The listing builds one solid part. Answer for the finished solid, in the listing's coordinates (mm). Face numbers are marked on the shaded views. A direction names the side the tool comes from. Coordinates: 2 decimals unless noted, no trailing zeros. Write each loop counter-clockwise with the first axis right and the second up, starting at its lowest first coordinate (ties: lowest second). Pieces come first, ordered by that corner, then holes.
(1) The part is cut by section A-A on y = 41.5. Determine the outline of the cut face in (x, z).
(2) Given P1, Ø4, axis at x = -15.5, z = -48.5, coming from the -Y side; P2, Ø16, axis at y = 49.5, z = -34.5, coming from the -X side; P3, Ø2, axis at x = 29, y = -26.5, coming from the -Z side, each flat-ended and moving along its own axis, determine where each tip first touches the part or whether it passes through.
(3) Which of the six approach directions +Z, -Z, +X, -X, +Y, -Y give full straight-line access (tool end or side, diameter ignored) to the marked faces 1 and 2?
(4) The part is cut by section B-B on z = -39. Determine the outline of the cut face in (x, y).
(5) Straight lines are drawn through the part: line 1 (Y direction, x = -22, z = -18); line 2 (Z direction, x = 11, y = -1). For each, find the intervals that lie inside material, in ascending order.
from build123d import *

# Parameters (mm, degrees)
EXTRUDE_1_DEPTH           = 3
CUT_EXTRUDE_10_DEPTH      = 76.423640864
CUT_EXTRUDE_10_DEPTH_BACK = 3
SKETCH_9_W                = 95.828885904
SKETCH_9_H                = 3
EXTRUDE_2_DEPTH           = 20
SKETCH_10_W               = 95.828885904
SKETCH_10_H               = 3
EXTRUDE_3_DEPTH           = 60


with BuildPart() as part:
    # 草图1 → 凸台-拉伸1 (new body)
    with BuildSketch(Plane.XY):
        with BuildLine():
            Line((-60, 34), (-60, -34))
            add(Edge.make_bspline(
                [(-60, -34), (0, -61.168399395), (60, -34)],
                knots=[0.841357477, 0.841357477, 0.841357477, 2.300235176, 2.300235176, 2.300235176], degree=2, weights=[1, 0.745548499, 1]))
            Line((60, -34), (60, 34))
            add(Edge.make_bspline(
                [(60, 34), (0, 61.168399395), (-60, 34)],
                knots=[3.982950131, 3.982950131, 3.982950131, 5.44182783, 5.44182783, 5.44182783], degree=2, weights=[1, 0.745548499, 1]))
        make_face()
    extrude(amount=EXTRUDE_1_DEPTH)

    # 草图7 → 切除-拉伸10 (cut, two sides: drawn at the far end of the back side and taken through both)
    with BuildSketch(Plane(origin=(0, 0, 0), x_dir=(-1, 0, 0), z_dir=(0, 0, -1)).offset(-CUT_EXTRUDE_10_DEPTH_BACK)):
        with BuildLine():
            Line((-47.914442952, 38.608895735), (-0.047490379, 38.608895735))
            Line((-0.047490379, 38.608895735), (47.914442952, 38.608895735))
            add(Edge.make_bspline(
                [(-47.914442952, 38.608895735), (0, 53.86648698), (47.914442952, 38.608895735)],
                knots=[4.161758339, 4.161758339, 4.161758339, 5.263019622, 5.263019622, 5.263019622], degree=2, weights=[0.945270908, 0.800277591, 0.945270908]))
        make_face()
    extrude(amount=CUT_EXTRUDE_10_DEPTH + CUT_EXTRUDE_10_DEPTH_BACK, mode=Mode.SUBTRACT)

    # 草图9 → 凸台-拉伸2 (add)
    with BuildSketch(Plane(origin=(0, 38.608895735, 0), x_dir=(1, 0, 0), z_dir=(0, 1, 0))):
        with Locations((0, -1.5)):
            Rectangle(SKETCH_9_W, SKETCH_9_H)
    extrude(amount=EXTRUDE_2_DEPTH)

    # 草图10 → 凸台-拉伸3 (add)
    with BuildSketch(Plane(origin=(0, 0, 0), x_dir=(-1, 0, 0), z_dir=(0, 0, -1))):
        with Locations((0, 57.108895735)):
            Rectangle(SKETCH_10_W, SKETCH_10_H)
    extrude(amount=EXTRUDE_3_DEPTH)


solid = part.part
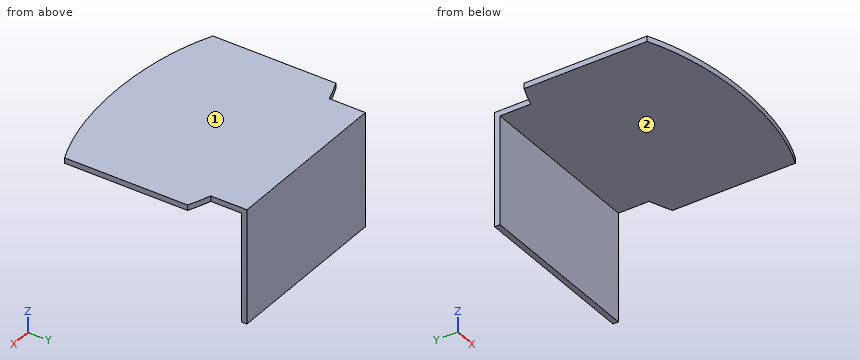
Model answer:
1. outline: (-47.91, 0) - (47.91, 0) - (47.91, 3) - (-47.91, 3) - close
2. P1: stops at y = 55.61
2. P2: stops at x = -47.91
2. P3: stops at z = 0
3. face 1: +Z, +X, -X, +Y, -Y
3. face 2: -Z, +X, -X, -Y
4. outline: (-47.91, 55.61) - (47.91, 55.61) - (47.91, 58.61) - (-47.91, 58.61) - close
5. line 1: y = 55.61 to 58.61
5. line 2: z = 0 to 3
